from build123d import *

# Parameters (mm, degrees)
F0_W     = 15.8369
F0_H     = 7.8486
F1_DEPTH = 9.5885
F2_R     = 2.4511
F4_DEPTH = 1.778
F3_R     = 2.4511
F5_DEPTH = 1.778
F6_W     = 14.351
F6_H     = 6.35
F8_DEPTH = 8.3312
F7_R     = 1.4859
F9_DEPTH = 8.3312


with BuildPart() as f1:
    # F0 (on Top) → F1 (new body)
    with BuildSketch(Plane.XY):
        Rectangle(F0_W, F0_H)
    extrude(amount=F1_DEPTH)

    # F2 (on face) → F4 (join)
    with BuildSketch(Plane.XY.offset(9.5885)):
        with Locations((-3.99415, 0)):
            Circle(F2_R)
    extrude(amount=F4_DEPTH)

    # F3 (on face) → F5 (join)
    with BuildSketch(Plane.XY.offset(9.5885)):
        with Locations((3.99415, 0)):
            Circle(F3_R)
    extrude(amount=F5_DEPTH)

    # F6 (on face) → F8 (cut)
    with BuildSketch(Plane(origin=(0, 0, 0), x_dir=(1, 0, 0), z_dir=(0, 0, -1))):
        Rectangle(F6_W, F6_H)
    extrude(amount=-F8_DEPTH, mode=Mode.SUBTRACT)

    # F7 (on face) → F9 (join)
    with BuildSketch(Plane(origin=(0, 0, 0), x_dir=(1, 0, 0), z_dir=(0, 0, -1))):
        Circle(F7_R)
    extrude(amount=-F9_DEPTH)


solid = f1.part
For this review, take the finished solid that the model builds, in its own axes (mm). A direction names the side the tool comes from. Round coordinates to 2 decimals unless told otherwise and drop trailing zeros. Loops run counter-clockwise (first coordinate to the right, second up) from the corner with the lowest first, then second, coordinate; pieces in that order, holes last. Notation, with made-up numbers: (70, -13) - (125, -13) arc R25 ccw to (125, 22) - close; hole circle Ø8 at (43, 61). An arc over 180 degrees is marked (long way). One line per question, with ' | ' between items.
Q1. Take a section at A-A (z = 3.25). Give the boundary of the cut face in (x, y) (1 decimal).
Taken from the geometry:
outline: (-7.9, -3.9) - (7.9, -3.9) - (7.9, 3.9) - (-7.9, 3.9) - close; circle Ø3 at (0, 0); hole (-7.2, -3.2) - (7.2, -3.2) - (7.2, 3.2) - (-7.2, 3.2) - close
Q2. The part is to be moulded in two halves that separate along X. For faces 4 (the flat face through (0, 0, 0)), 5 (the flat face through (-7.918, 0, 5)), 6 (the cylindrical face through (1.545, 0.108, 10.465)), 7 (the flat face through (0, 3.175, 4)), say which applies: released by +X, released by -X, zero draft, split by the parting line, or undercut.
Taken from the geometry:
face 4: zero draft | face 5: released by -X | face 6: undercut | face 7: undercut
Q3. Tool access review of faces 1 (the flat face through (0, 0, 9.588)), 2 (the flat face through (-7.176, 0, 4)), 3 (the flat face through (4, 0, 11.366)): name each direction out of +Z, -Z, +X, -X, +Y, -Y from which nothing blocks a thin tool from reaching the whole face with its end or side.
Taken from the geometry:
face 1: +Z | face 2: -Z | face 3: +Z, +X, -X, +Y, -Y
Q4. For line 1 along Y through (x, z) = (7, 4.25) (3 decimals); line 2 along X through (y, z) = (-2.25, 0.5); line 3 along X through (y, z) = (-0.5, 8), list the stretches that pass through material, from the lowest coordinate up. Write a range as [from, to].
Taken from the geometry:
line 1: y = [-3.924, -3.175], [3.175, 3.924] | line 2: x = [-7.92, -7.18], [7.18, 7.92] | line 3: x = [-7.92, -7.18], [-1.4, 1.4], [7.18, 7.92]
Q5. Take a section at D-D (x = 0). Give the boundary of the cut face in (y, z) (1 decimal).
Taken from the geometry:
outline: (-3.9, 0) - (-3.2, 0) - (-3.2, 8.3) - (-1.5, 8.3) - (-1.5, 0) - (1.5, 0) - (1.5, 8.3) - (3.2, 8.3) - (3.2, 0) - (3.9, 0) - (3.9, 9.6) - (-3.9, 9.6) - close
Q6. For pin 1 (1 mm diameter, centred on x = 4.5, y = 1, fed in from -Z), flat-tipped, find the tip position at first contact; note if it passes through.
Taken from the geometry:
pin 1: stops at z = 8.33
Q7. Take a section at B-B (x = 7). Give the boundary of the cut face in (y, z) (1 decimal), and give its area (3 significant figures).
Taken from the geometry:
outline: (-3.9, 0) - (-3.2, 0) - (-3.2, 8.3) - (3.2, 8.3) - (3.2, 0) - (3.9, 0) - (3.9, 9.6) - (-3.9, 9.6) - close | area: 22.4 mm²
Q8. Take a section at C-C (y = 0). Give the boundary of the cut face in (x, z).
Taken from the geometry:
outline: (-7.92, 0) - (-7.18, 0) - (-7.18, 8.33) - (-1.49, 8.33) - (-1.49, 0) - (1.49, 0) - (1.49, 8.33) - (7.18, 8.33) - (7.18, 0) - (7.92, 0) - (7.92, 9.59) - (6.45, 9.59) - (6.45, 11.37) - (1.54, 11.37) - (1.54, 9.59) - (-1.54, 9.59) - (-1.54, 11.37) - (-6.45, 11.37) - (-6.45, 9.59) - (-7.92, 9.59) - close
